Work out the finished part from the listing and answer in its coordinate system (mm). Coordinates: 2 decimals unless noted, no trailing zeros. Write each loop counter-clockwise with the first axis right and the second up, starting at its lowest first coordinate (ties: lowest second). Pieces come first, ordered by that corner, then holes. Notation, with made-up numbers: (-10, -34) - (-6, -34) arc R5 cw to (-6, -26) - close; hole circle Ø11 at (1.25, 75.25). An arc over 180 degrees is marked (long way). Use a Markdown table: item, result. Add a question column.
(1) For a pull along Z with two mould halves and no side action, classify faces 1 (the face through (-38, 2, 0)), 2 (the face through (-25.4, 2, -38)), 3 (the face through (-51, 2, -25.4)), 4 (the face through (-35.72, 1.57, -12.8)) as released by +Z, released by -Z, zero draft, split by the parting line, or undercut.
(2) The part is cut by section C-C, the plane z = -38.1. Give the vertices of the cut face in (x, y) (3 decimals), then the cut area to 3 significant figures.
(3) Find the intervals of material crossed by line 1 (X direction, y = 2.2, z = -38.1); line 2 (X direction, y = 0.65, z = -13), in increasing order. Write a range as from..to.
(4) The part is cut by section A-A, the plane x = -63.5. Give the vertices of the cut face in (y, z) (3 decimals), then the cut area to 3 significant figures.
(5) The part is cut by section B-B, the plane y = 1.1. Give the vertices of the cut face in (x, z).
(6) The part is cut by section D-D, the plane x = -12.7. Give the vertices of the cut face in (y, z) (3 decimals), then the cut area to 3 significant figures.
(7) Given pin 1 Ø10 at (x, z) = (-26, -44.5) entering from +Y (3 decimals); pin 2 Ø1.6 at (x, y) = (-51.5, 1.5) entering from -Z, each flat-ended and moving along its own axis, determine where each tip first touches the part or whether it passes through.
Autodesk Inventor part; units mm, degrees
ref_plane "YZ Plane" through (0, 0, 0) normal (1, 0, 0) x (0, 1, 0)
ref_plane "XZ Plane" through (0, 0, 0) normal (0, 1, 0) x (-1, 0, 0)
ref_plane "XY Plane" through (0, 0, 0) normal (0, 0, 1) x (1, 0, 0)
sketch "Sketch1" plane through (0, 0, 0) normal (0, 1, 0) x (-1, 0, 0)
  line L0 (0, 0) -> (76.2, 0)
  line L1 (76.2, 0) -> (76.2, -25.4)
  line L2 (76.2, -25.4) -> (25.4, -25.4)
  line L3 (25.4, -25.4) -> (25.4, -50.8)
  line L4 (25.4, -50.8) -> (0, -50.8)
  line L5 (0, -50.8) -> (0, 0)
  line L6 (0, 0) -> (0, -12.7)
  line L7 (0, -12.7) -> (12.7, -12.7)
  circle A0 centre (12.7, -12.7) radius 2.3813
  line L8 (12.7, -12.7) -> (12.7, -38.1)
  circle A1 centre (12.7, -38.1) radius 2.3812
  line L9 (12.7, -12.7) -> (38.1, -12.7)
  circle A2 centre (38.1, -12.7) radius 2.3812
  line L10 (38.1, -12.7) -> (63.5, -12.7)
  circle A3 centre (63.5, -12.7) radius 2.3813
  dimension "d9" = 76.2
  dimension "d10" = 25.4
  dimension "d11" = 50.8
  dimension "d12" = 25.4
  dimension "d13" = 25.4
  dimension "d14" = 50.8
  dimension "d15" = 12.7
  dimension "d16" = 12.7
  dimension "d17" = 4.7625
  dimension "d18" = 25.4
  dimension "d19" = 4.7625
  dimension "d20" = 25.4
  dimension "d21" = 4.7625
  dimension "d22" = 25.4
  dimension "d23" = 4.7625
extrude "Extrusion1" add sketch "Sketch1" along normal blind 3.175
properties part number "LPlate"
Model answer:
| question | item | result |
|---|---|---|
| 1 | face 1 | released by +Z |
| 1 | face 2 | zero draft |
| 1 | face 3 | released by -Z |
| 1 | face 4 | undercut |
| 2 | outline | (-25.4, 0) - (-15.081, 0) - (-15.081, 3.175) - (-25.4, 3.175) - close; (-10.319, 0) - (0, 0) - (0, 3.175) - (-10.319, 3.175) - close |
| 2 | area | 65.5 mm^2 |
| 3 | line 1 | -25.4..-15.08, -10.32..0 |
| 3 | line 2 | -76.2..-65.86, -61.14..-40.46, -35.74..-15.06, -10.34..0 |
| 4 | outline | (0, -25.4) - (3.175, -25.4) - (3.175, -15.081) - (0, -15.081) - close; (0, -10.319) - (3.175, -10.319) - (3.175, 0) - (0, 0) - close |
| 4 | area | 65.5 mm^2 |
| 5 | outline | (-76.2, -25.4) - (-25.4, -25.4) - (-25.4, -50.8) - (0, -50.8) - (0, 0) - (-76.2, 0) - close; hole circle Ø4.76 at (-63.5, -12.7); hole circle Ø4.76 at (-38.1, -12.7); hole circle Ø4.76 at (-12.7, -38.1); hole circle Ø4.76 at (-12.7, -12.7) |
| 6 | outline | (0, -50.8) - (3.175, -50.8) - (3.175, -40.481) - (0, -40.481) - close; (0, -35.719) - (3.175, -35.719) - (3.175, -15.081) - (0, -15.081) - close; (0, -10.319) - (3.175, -10.319) - (3.175, 0) - (0, 0) - close |
| 6 | area | 131 mm^2 |
| 7 | pin 1 | y = 3.175 |
| 7 | pin 2 | z = -25.4 |
